Geometry: final body of the model. Coordinates: model frame, mm. A direction names the side the tool comes from. Round coordinates to 2 decimals unless told otherwise and drop trailing zeros. Write each loop counter-clockwise with the first axis right and the second up, starting at its lowest first coordinate (ties: lowest second). Pieces come first, ordered by that corner, then holes. Notation, with made-up numbers: M -9.5,67 L 38.5,67 A19 ccw 38.5,75 Z; hole C 52.5,-25.75 d11. An arc over 180 degrees is marked long. Put each result on its own line as item: value. Start each with the question number.
Autodesk Inventor part; units mm, degrees
ref_plane "YZ Plane" through (0, 0, 0) normal (1, 0, 0) x (0, 1, 0)
ref_plane "XZ Plane" through (0, 0, 0) normal (0, 1, 0) x (-1, 0, 0)
ref_plane "XY Plane" through (0, 0, 0) normal (0, 0, 1) x (1, 0, 0)
sketch "Sketch1" plane through (0, 0, 0) normal (0, 1, 0) x (-1, 0, 0)
  circle A0 centre (0, 0) radius 4.1275
  line L0 (7.3152, 7.3152) -> (-7.3152, 7.3152)
  line L1 (-7.3152, 7.3152) -> (-7.3152, -7.3025)
  line L2 (-7.3152, -7.3025) -> (7.3152, -7.3025)
  line L3 (7.3152, -7.3025) -> (7.3152, 7.3152)
  line L4 (7.3152, 20.0152) -> (-7.3152, 20.0152)
  line L5 (-7.3152, 20.0152) -> (-7.3152, -20.0025)
  line L6 (-7.3152, -20.0025) -> (7.3152, -20.0025)
  line L7 (7.3152, -20.0025) -> (7.3152, 20.0152)
  circle A1 centre (0, 13.6652) radius 2.159
  circle A2 centre (0, -13.6525) radius 2.159
  line L8 (7.3152, 7.3152) -> (20.0152, 7.3152)
  line L9 (20.0152, 7.3152) -> (20.0152, -7.3025)
  line L10 (20.0152, -7.3025) -> (7.3152, -7.3025)
  line L11 (7.3152, -7.3025) -> (7.3152, 7.3152)
  line L12 (-7.3152, 7.3152) -> (-20.0152, 7.3152)
  line L13 (-20.0152, 7.3152) -> (-20.0152, -7.3025)
  line L14 (-20.0152, -7.3025) -> (-7.3152, -7.3025)
  line L15 (-7.3152, -7.3025) -> (-7.3152, 7.3152)
  circle A3 centre (13.6652, 0.0063) radius 1.9812
  circle A4 centre (-13.6652, 0.0063) radius 1.9812
  point P0 (-7.3152, 7.3152)
  point P1 (-7.3152, -7.3025)
  point P2 (-7.3152, -7.3025)
  dimension "d0" = 8.255
  dimension "d1" = 7.3025
  dimension "d2" = 7.3152
  dimension "d3" = 7.3152
  dimension "d4" = 7.3152
  dimension "d5" = 4.318
  dimension "d6" = 4.318
  dimension "d7" = 12.7
  dimension "d8" = 12.7
  dimension "d9" = 6.35
  dimension "d10" = 6.35
  dimension "d23" = 12.7
  dimension "d24" = 12.7
  dimension "d25" = 3.9624
  dimension "d26" = 3.9624
extrude "Extrusion1" add sketch "Sketch1" along normal blind 12.7 contours L3 L2 L1 L0 | L0 L5 L4 L7 | L7 L6 L5 L2
extrude "Extrusion3" add sketch "Sketch1" along normal blind 3.81 contours A0
fillet "Fillet5" radius 1.778 2 edges at (0, 12.7, 20.0152) (0, 12.7, -20.0025)
chamfer "Chamfer2" distance 2.286 angle 45 2 edges at (2.159, 12.7, 13.6652) (2.159, 12.7, -13.6525)
properties part number "Rod Holder Top V1_3DPrint"
1) Draft query along Z for faces 3 (the face through (-1.062, 10.557, -15.695)), 4 (the face through (-0.1, 12.19, -19.47)), 5 (the face through (0, 0, 0)). Return one class per face: +Z half, -Z half, draft (parallel to the pull), parting line (faces both ways), or undercut.
2) Section A-A, the plane x = 0. Output: boundary loops of the cut face in (y, z), and give its area (3 significant figures).
3) First-contact query: pin 1 (3.5 mm diameter, centred on x = 0, z = 13.67, fed in from -Y); pin 2 (5.5 mm diameter, centred on x = 0, z = -13.65, fed in from +Y). Flat tips, straight axial feed; report the tip coordinate or a pass-through.
4) Ray query, probe 1 along Z at (x, y) = (0, 7); probe 2 along Z at (x, y) = (-0.75, 2); probe 3 along X at (y, z) = (0.5, -13.5). Return the intervals inside material, ascending.
5) Access query for faces 1 (the face through (-3.937, 8.193, -1.24)), 2 (the face through (0.102, 12.193, 19.481)). Directions: +Z, -Z, +X, -X, +Y, -Y. A direction counts if a zero-diameter tool reaches every point of the face in a straight line with its end or side. Return the directions, or none.
6) Section C-C, the plane y = 9.75. Output: boundary loops of the cut face in (x, z) (1 decimal).
7) Section B-B, the plane z = 0. Output: boundary loops of the cut face in (x, y), and give its area (3 significant figures).
Solved:
1. face 3: undercut
1. face 4: -Z half
1. face 5: draft
2. outline: M 0,-20 L 10.92,-20 A1.78 ccw 12.7,-18.22 L 12.7,-18.1 L 10.41,-15.81 L 0,-15.81 Z; M 0,-11.49 L 10.41,-11.49 L 12.7,-9.21 L 12.7,-4.13 L 3.81,-4.13 L 3.81,4.13 L 12.7,4.13 L 12.7,9.22 L 10.41,11.51 L 0,11.51 Z; M 0,15.82 L 10.41,15.82 L 12.7,18.11 L 12.7,18.24 A1.78 ccw 10.92,20.02 L 0,20.02 Z
2. area: 313 mm2
3. pin 1: passes through
3. pin 2: stops at y = 11.01
4. probe 1: z = -20 to -15.81, -11.49 to -4.13, 4.13 to 11.51, 15.82 to 20.02
4. probe 2: z = -20 to -15.68, -11.63 to 11.64, 15.69 to 20.02
4. probe 3: x = -7.32 to -2.15, 2.15 to 7.32
5. face 1: +Y
5. face 2: +Z, +X, -X, +Y
6. outline: M -7.3,-20 L 7.3,-20 L 7.3,20 L -7.3,20 Z; hole C 0,0 d8.3; hole C 0,-13.7 d4.3; hole C 0,13.7 d4.3
7. outline: M -7.32,0 L 7.32,0 L 7.32,12.7 L 4.13,12.7 L 4.13,3.81 L -4.13,3.81 L -4.13,12.7 L -7.32,12.7 Z
7. area: 112 mm2
